Source: CAD feature listing. Evaluate the final solid. Frame: model axes, mm. Face numbers are marked on the shaded views. A direction names the side the tool comes from. Round coordinates to 2 decimals unless told otherwise and drop trailing zeros. Loops run counter-clockwise (first coordinate to the right, second up) from the corner with the lowest first, then second, coordinate; pieces in that order, holes last. Notation, with made-up numbers: M 39.25,-16 L 83.25,-16 A35 ccw 83.25,22 Z; hole C -26.5,54 d2. An arc over 180 degrees is marked long. One line per item, written item: value.
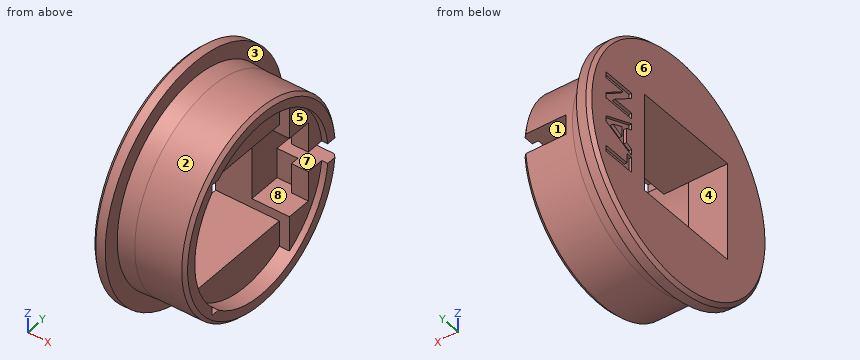
from build123d import *

# Parameters (mm, degrees)
SKIZZE2_W                       = 14.75
SKIZZE2_H                       = 16.35
SCHNITT_LINEAR_AUSTRAGEN1_DEPTH = 28.461063344
AUFSATZ_LINEAR_AUSTRAGEN1_DEPTH = 3.9
AUFSATZ_LINEAR_AUSTRAGEN2_DEPTH = 9.1
SCHNITT_LINEAR_AUSTRAGEN2_DEPTH = 6
AUFSATZ_LINEAR_AUSTRAGEN3_DEPTH = 7.6
FASE1_SIZE                      = 0.5
SCHNITT_LINEAR_AUSTRAGEN3_DEPTH = 0.4
SCHNITT_LINEAR_AUSTRAGEN4_REACH = 29.461
SKIZZE13_W                      = 20
SKIZZE13_H                      = 1.212730801
SCHNITT_LINEAR_AUSTRAGEN6_DEPTH = 2.4


with BuildPart() as part:
    # Skizze1 → Rotation1 (revolve)
    with BuildSketch(Plane(origin=(0, 0, 0), x_dir=(1, 0, 0), z_dir=(0, 1, 0)), mode=Mode.PRIVATE) as rotation1_sk:
        Polygon((0, 0), (0, 17.5), (1.9, 17.5), (1.9, 15), (11.9, 15), (11.9, 13.1), (1.9, 13.1), (1.9, 0), align=None)
    revolve(rotation1_sk.sketch.rotate(Axis((-3.369811321, 0, 0), (1, 0, 0)), 180), axis=Axis((-3.369811321, 0, 0), (1, 0, 0)))

    # Skizze2 → Schnitt-Linear austragen1 (cut, through all)
    with BuildSketch(Plane.ZY):
        with Locations((0, -1.5)):
            Rectangle(SKIZZE2_W, SKIZZE2_H)
    extrude(amount=-SCHNITT_LINEAR_AUSTRAGEN1_DEPTH, mode=Mode.SUBTRACT)

    # Skizze3 → Aufsatz-Linear austragen1 (add)
    with BuildSketch(Plane(origin=(1.9, 0, 0), x_dir=(0, 0, -1), z_dir=(1, 0, 0))):
        with BuildLine():
            Line((-8.832008548, -9.675), (8.832008548, -9.675))
            ThreePointArc((8.832008548, -9.675), (0, -13.1), (-8.832008548, -9.675))
        make_face()
    extrude(amount=AUFSATZ_LINEAR_AUSTRAGEN1_DEPTH)

    # Skizze4 → Aufsatz-Linear austragen2 (add)
    with BuildSketch(Plane(origin=(1.9, 0, 0), x_dir=(0, 0, -1), z_dir=(1, 0, 0))):
        with BuildLine():
            Line((-11.271839912, 6.675), (11.271839912, 6.675))
            ThreePointArc((11.271839912, 6.675), (0, 13.1), (-11.271839912, 6.675))
        make_face()
    extrude(amount=AUFSATZ_LINEAR_AUSTRAGEN2_DEPTH)

    # Skizze6 → Schnitt-Linear austragen2 (cut, symmetric)
    with BuildSketch(Plane.XY):
        Polygon((5.4, 6.675), (5.4, 11.625), (8.5, 11.625), (8.5, 10.375), (11, 10.375), (11, 6.675), align=None)
    extrude(amount=SCHNITT_LINEAR_AUSTRAGEN2_DEPTH, both=True, mode=Mode.SUBTRACT)

    # Skizze7 → Aufsatz-Linear austragen3 (add)
    with BuildSketch(Plane(origin=(1.9, 0, 0), x_dir=(0, 0, -1), z_dir=(1, 0, 0))):
        with BuildLine():
            Line((-11.271839912, 6.675), (-7.375, 6.675))
            Line((-7.375, 6.675), (-7.375, -9.675))
            Line((-7.375, -9.675), (-8.832008548, -9.675))
            ThreePointArc((-8.832008548, -9.675), (-12.956535252, -1.933441044), (-11.271839912, 6.675))
        make_face()
        with BuildLine():
            Line((7.375, 6.675), (7.375, -9.675))
            Line((7.375, -9.675), (8.832008548, -9.675))
            ThreePointArc((8.832008548, -9.675), (12.956535252, -1.933441044), (11.271839912, 6.675))
            Line((11.271839912, 6.675), (7.375, 6.675))
        make_face()
    extrude(amount=AUFSATZ_LINEAR_AUSTRAGEN3_DEPTH)

    # Fase1
    fase1_edges = [part.edges().sort_by_distance(p)[0] for p in [
        (11.9, 0, -15),
        (0, 0, -17.5),
    ]]
    chamfer(fase1_edges, length=FASE1_SIZE)

    # Skizze8 → Schnitt-Linear austragen3 (cut)
    # profile 1 of 3: a face of its own
    with BuildSketch(Plane.ZY):
        Polygon((-6.298076923, 14.175), (-5.400641026, 14.175), (-5.400641026, 10.072435897), (-3.990384615, 10.072435897), (-3.990384615, 9.175), (-6.298076923, 9.175), align=None)
    # profile 2 of 3: a face of its own
    with BuildSketch(Plane.ZY):
        Polygon((-1.681690705, 14.175), (-0.849358974, 14.175), (1.169871795, 9.175), (0.211338141, 9.175), (-0.177283654, 10.200641026), (-2.355769231, 10.200641026), (-2.744391026, 9.175), (-3.701923077, 9.175), align=None)
        Polygon((-1.266025641, 12.833854167), (-2.015224359, 11.098076923), (-0.516826923, 11.098076923), align=None, mode=Mode.SUBTRACT)
    # profile 3 of 3: a face of its own
    with BuildSketch(Plane.ZY):
        Polygon((1.907051282, 14.175), (2.715344551, 14.175), (4.983974359, 10.884735577), (4.983974359, 14.175), (5.881410256, 14.175), (5.881410256, 9.175), (5.067107372, 9.175), (2.804487179, 12.455248397), (2.804487179, 9.175), (1.907051282, 9.175), align=None)
    extrude(amount=-SCHNITT_LINEAR_AUSTRAGEN3_DEPTH, mode=Mode.SUBTRACT)

    # Schnitt-Linear austragen4: up to this face of the body (flat: up to its plane)
    schnitt_linear_austragen4_end = Plane(part.part.faces().sort_by_distance((5.4, 9.15, 0))[0])
    # Skizze10 → Schnitt-Linear austragen4 (cut, up to the picked face)
    with BuildSketch(Plane(origin=(11.9, 0, 0), x_dir=(0, 0, -1), z_dir=(1, 0, 0)), mode=Mode.PRIVATE) as schnitt_linear_austragen4_sk1:
        with BuildLine():
            Line((-1.5, 10.375), (-1.5, 14.924811557))
            ThreePointArc((-1.5, 14.924811557), (0, 15), (1.5, 14.924811557))
            Line((1.5, 14.924811557), (1.5, 10.375))
            Line((1.5, 10.375), (-1.5, 10.375))
        make_face()
    schnitt_linear_austragen4_tool1 = split(extrude(schnitt_linear_austragen4_sk1.sketch, amount=-SCHNITT_LINEAR_AUSTRAGEN4_REACH, mode=Mode.PRIVATE), bisect_by=schnitt_linear_austragen4_end, keep=Keep.BOTH, mode=Mode.PRIVATE)
    add(schnitt_linear_austragen4_tool1.solids().sort_by(Axis((11.9, 12.675036, 0), (-1, 0, 0)))[0], mode=Mode.SUBTRACT)

    # Skizze13 → Schnitt-Linear austragen6 (cut)
    with BuildSketch(Plane(origin=(11.9, 0, 0), x_dir=(0, 0, -1), z_dir=(1, 0, 0))):
        with Locations((0, -9.0686346)):
            Rectangle(SKIZZE13_W, SKIZZE13_H)
    extrude(amount=-SCHNITT_LINEAR_AUSTRAGEN6_DEPTH, mode=Mode.SUBTRACT)

    # Skizze14 → Rotation2 (revolve)
    with BuildSketch(Plane.XY, mode=Mode.PRIVATE) as rotation2_sk:
        Polygon((4.4, 15), (1.9, 15.15), (1.9, 15), align=None)
    revolve(rotation2_sk.sketch.rotate(Axis((-3.369811321, 0, 0), (-1, 0, 0)), 90), axis=Axis((-3.369811321, 0, 0), (-1, 0, 0)))


solid = part.part
1. Reachability of the marked faces 4, 5, 6, 7 and 8 from +Z, -Z, +X, -X, +Y, -Y: full face, straight path, thin tool, end or side. Return the list, or none.
Report:
face 4: +X, -X
face 5: +X
face 6: +Z, -Z, -X, +Y, -Y
face 7: +X, +Y
face 8: none
2. Pull-direction query (Z, two-part tool) for the marked faces 1, 2 and 3; classes: released by +Z, released by -Z, zero draft, split by the parting line, or undercut.
Report:
face 1: undercut
face 2: split by the parting line
face 3: zero draft
3. Pin query (flat end, axial travel): pin 1 (4 mm diameter, centred on x = 10.5, z = -14, fed in from +Y); pin 2 (1.5 mm diameter, centred on x = 9, y = 9, fed in from +Z); pin 3 (0.8 mm diameter, centred on x = 9.5, z = 3.5, fed in from -Y). Return the tip coordinate at first contact, or that it passes through.
Report:
pin 1: stops at y = 9
pin 2: stops at z = 12.53
pin 3: stops at y = -14.68
4. Ray query, line 1 (Y direction, x = 7.5, z = 2.5) (3 decimals); line 2 (Y direction, x = 10, z = -12); line 3 (X direction, y = -9, z = -8). Return the intervals inside material, ascending. Write a range as [from, to].
Report:
line 1: y = [-14.79, -12.859], [11.625, 14.79]
line 2: y = [-9, -5.25], [5.25, 9]
line 3: x = [0, 9.5]
5. Section query B-B (x = 3). Return the cut outline in (y, z) (3 decimals).
Report:
outline: C 0,0 d30.168; hole M -9.675,-7.375 L 6.675,-7.375 L 6.675,7.375 L -9.675,7.375 Z
6. Section query A-A (y = 0). Return the cut outline in (x, z) (3 decimals), and give its area (3 significant figures).
Report:
outline: M 0,-17 L 0.5,-17.5 L 1.9,-17.5 L 1.9,-15.15 L 4.4,-15 L 11.4,-15 L 11.9,-14.5 L 11.9,-13.1 L 9.5,-13.1 L 9.5,-7.375 L 0,-7.375 Z; M 0,7.375 L 9.5,7.375 L 9.5,13.1 L 11.9,13.1 L 11.9,14.5 L 11.4,15 L 4.4,15 L 1.9,15.15 L 1.9,17.5 L 0.5,17.5 L 0,17 Z
area: 163 mm2
